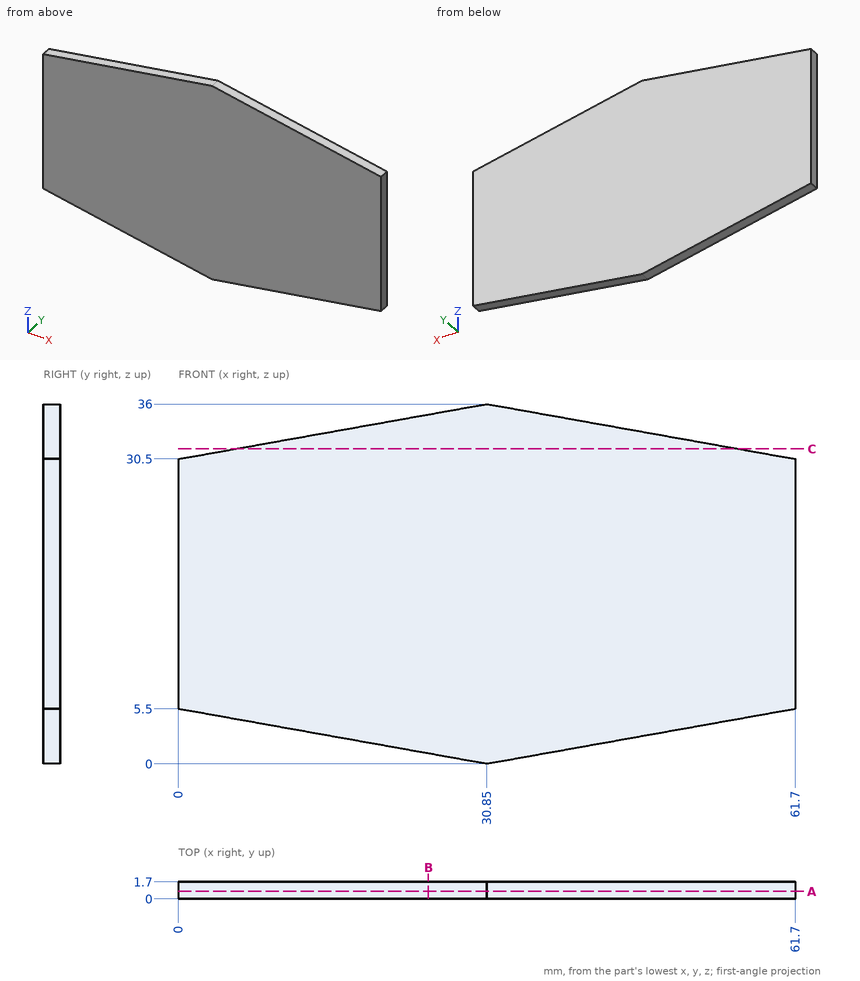
The figure shows three views and two pictorial views of one solid part (mm, origin at its lowest corner). Answer the questions. Round coordinates to 2 decimals unless told otherwise and drop trailing zeros. Loops run counter-clockwise (first coordinate to the right, second up) from the corner with the lowest first, then second, coordinate; pieces in that order, holes last. Notation, with made-up numbers: M -33,44 L 20,44 A13 ccw 20,62 Z; hole C 0.5,83 d5. An arc over 180 degrees is marked long. Return JSON: item names as keys, results as strings.
Q1. Find section C-C, the plane z = 31.5. Determine the outline of the cut face in (x, y).
Results list:
{"outline": "M 5.61,0 L 56.09,0 L 56.09,1.7 L 5.61,1.7 Z"}
Q2. Find section A-A, the plane y = 0.75. Determine the outline of the cut face in (x, z).
Results list:
{"outline": "M 0,5.5 L 30.85,0 L 61.7,5.5 L 61.7,30.5 L 30.85,36 L 0,30.5 Z"}
Q3. Find the intervals of material crossed by line 1 along Z through (x, y) = (59, 0.85); line 2 along Z through (x, y) = (23, 1.2), in increasing order. Write a range as from..to.
Results list:
{"line 1": "z = 5.02..30.98", "line 2": "z = 1.4..34.6"}
Q4. Each of these flat-tipped pins is pushed along its axis until it touches: pin 1 Ø1 at (x, y) = (32.5, 0.5) entering from +Z (3 decimals); pin 2 Ø1 at (x, y) = (21, 1.5) entering from +Z. Where does it stop, or does it pass through?
Results list:
{"pin 1": "stops at z = 35.795", "pin 2": "stops at z = 34.33"}
Q5. Find section B-B, the plane x = 25. Determine the outline of the cut face in (y, z).
Results list:
{"outline": "M 0,1.04 L 1.7,1.04 L 1.7,34.96 L 0,34.96 Z"}
